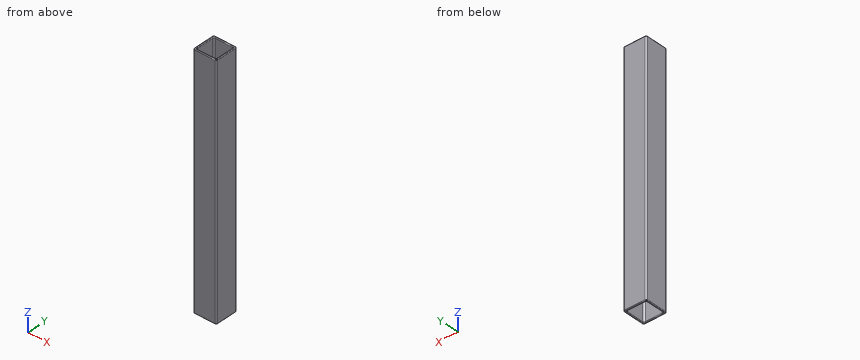
from build123d import *

# Parameters (mm, degrees)
BOSS_EXTRUDE1_DEPTH = 397
BOSS_EXTRUDE2_START = 0.678713738
BOSS_EXTRUDE2_DEPTH = 0.678713738
FILLET1_R           = 1


with BuildPart() as part:
    # Sketch1 → Boss-Extrude1 (new body)
    with BuildSketch(Plane.XY):
        with BuildLine():
            Line((2.54, 0), (35.56, 0))
            ThreePointArc((35.56, 0), (37.356051224, -0.743948776), (38.1, -2.54))
            Line((38.1, -2.54), (38.1, -35.56))
            ThreePointArc((38.1, -35.56), (37.356051224, -37.356051224), (35.56, -38.1))
            Line((35.56, -38.1), (2.54, -38.1))
            ThreePointArc((2.54, -38.1), (0.743948776, -37.356051224), (0, -35.56))
            Line((0, -35.56), (0, -2.54))
            ThreePointArc((0, -2.54), (0.743948776, -0.743948776), (2.54, 0))
        make_face()
        with BuildLine():
            Line((5.3086, -2.7686), (32.7914, -2.7686))
            ThreePointArc((32.7914, -2.7686), (34.587451224, -3.512548776), (35.3314, -5.3086))
            Line((35.3314, -5.3086), (35.3314, -32.7914))
            ThreePointArc((35.3314, -32.7914), (34.587451224, -34.587451224), (32.7914, -35.3314))
            Line((32.7914, -35.3314), (5.3086, -35.3314))
            ThreePointArc((5.3086, -35.3314), (3.512548776, -34.587451224), (2.7686, -32.7914))
            Line((2.7686, -32.7914), (2.7686, -5.3086))
            ThreePointArc((2.7686, -5.3086), (3.512548776, -3.512548776), (5.3086, -2.7686))
        make_face(mode=Mode.SUBTRACT)
    extrude(amount=BOSS_EXTRUDE1_DEPTH)

    # Sketch2 → Boss-Extrude2 (add)
    with BuildSketch(Plane(origin=(0, 0, 0), x_dir=(-1, 0, 0), z_dir=(0, 0, -1)).offset(BOSS_EXTRUDE2_START)):
        with BuildLine():
            Line((0, -35.56), (0, -2.54))
            ThreePointArc((0, -2.54), (-0.743948776, -0.743948776), (-2.54, 0))
            Line((-2.54, 0), (-35.56, 0))
            ThreePointArc((-35.56, 0), (-37.356051224, -0.743948776), (-38.1, -2.54))
            Line((-38.1, -2.54), (-38.1, -35.56))
            ThreePointArc((-38.1, -35.56), (-37.356051224, -37.356051224), (-35.56, -38.1))
            Line((-35.56, -38.1), (-2.54, -38.1))
            ThreePointArc((-2.54, -38.1), (-0.743948776, -37.356051224), (0, -35.56))
        make_face()
        with BuildLine():
            Line((-32.7914, -2.7686), (-5.3086, -2.7686))
            ThreePointArc((-5.3086, -2.7686), (-3.512548776, -3.512548776), (-2.7686, -5.3086))
            Line((-2.7686, -5.3086), (-2.7686, -32.7914))
            ThreePointArc((-2.7686, -32.7914), (-3.512548776, -34.587451224), (-5.3086, -35.3314))
            Line((-5.3086, -35.3314), (-32.7914, -35.3314))
            ThreePointArc((-32.7914, -35.3314), (-34.587451224, -34.587451224), (-35.3314, -32.7914))
            Line((-35.3314, -32.7914), (-35.3314, -5.3086))
            ThreePointArc((-35.3314, -5.3086), (-34.587451224, -3.512548776), (-32.7914, -2.7686))
        make_face(mode=Mode.SUBTRACT)
    extrude(amount=-BOSS_EXTRUDE2_DEPTH)

    # Fillet1
    fillet1_edges = [part.edges().sort_by_distance(p)[0] for p in [
        (37.356051224, -37.356051224, 397),
        (38.1, -19.05, 397),
        (37.356051224, -0.743948776, 397),
        (19.05, 0, 397),
        (0.743948776, -0.743948776, 397),
        (0, -19.05, 397),
        (3.512548776, -34.587451224, 397),
        (19.05, -35.3314, 397),
        (34.587451224, -34.587451224, 397),
        (35.3314, -19.05, 397),
        (34.587451224, -3.512548776, 397),
        (19.05, -2.7686, 397),
        (3.512548776, -3.512548776, 397),
        (2.7686, -19.05, 397),
        (0.743948776, -37.356051224, 397),
        (19.05, -2.7686, -0.678713738),
        (3.512548776, -3.512548776, -0.678713738),
        (2.7686, -19.05, -0.678713738),
        (3.512548776, -34.587451224, -0.678713738),
        (19.05, -35.3314, -0.678713738),
        (34.587451224, -34.587451224, -0.678713738),
        (35.3314, -19.05, -0.678713738),
        (34.587451224, -3.512548776, -0.678713738),
        (19.05, -38.1, -0.678713738),
        (0.743948776, -37.356051224, -0.678713738),
        (0, -19.05, -0.678713738),
        (0.743948776, -0.743948776, -0.678713738),
        (19.05, 0, -0.678713738),
        (37.356051224, -0.743948776, -0.678713738),
        (38.1, -19.05, -0.678713738),
        (37.356051224, -37.356051224, -0.678713738),
        (19.05, -38.1, 397),
    ]]
    fillet(fillet1_edges, radius=FILLET1_R)


solid = part.part
Work out the finished part from the listing and answer in its coordinate system (mm). Round coordinates to 2 decimals unless told otherwise and drop trailing zeros. Write each loop counter-clockwise with the first axis right and the second up, starting at its lowest first coordinate (ties: lowest second). Pieces come first, ordered by that corner, then holes. Notation, with made-up numbers: (20.5, 78.25) - (68.5, 78.25) arc R29 cw to (68.5, 114.25) - close; hole circle Ø11 at (24.25, 36.25). An arc over 180 degrees is marked (long way). Answer in a Markdown table with one row per item. Add a question column.
1. A cutting plane is placed at C-C, the plane x = 29.5. Determine the outline of the cut face in (y, z).
2. A cutting plane is placed at B-B, the plane z = 348.5. Determine the outline of the cut face in (x, y).
3. A cutting plane is placed at A-A, the plane y = -25.5. Determine the outline of the cut face in (x, z).
4. Find the intervals of material crossed by line 1 along X through (y, z) = (-8, 304); line 2 along Y through (x, z) = (9.5, 131); line 3 along Z through (x, y) = (2, -11), in increasing order. Write a range as from..to.
5. Given pin 1 (8 mm diameter, centred on x = 15.5, y = -7.5, fed in from +Z), flat-ended and moving along its own axis, determine where the tip first touches the part or whether it passes through.
Worked out:
| question | item | result |
|---|---|---|
| 1 | outline | (-38.1, 0.32) arc R1 ccw to (-37.1, -0.68) - (-36.33, -0.68) arc R1 ccw to (-35.33, 0.32) - (-35.33, 396) arc R1 ccw to (-36.33, 397) - (-37.1, 397) arc R1 ccw to (-38.1, 396) - close; (-2.77, 0.32) arc R1 ccw to (-1.77, -0.68) - (-1, -0.68) arc R1 ccw to (0, 0.32) - (0, 396) arc R1 ccw to (-1, 397) - (-1.77, 397) arc R1 ccw to (-2.77, 396) - close |
| 2 | outline | (0, -35.56) arc R2.54 ccw to (2.54, -38.1) - (35.56, -38.1) arc R2.54 ccw to (38.1, -35.56) - (38.1, -2.54) arc R2.54 ccw to (35.56, 0) - (2.54, 0) arc R2.54 ccw to (0, -2.54) - close; hole (2.77, -32.79) arc R2.54 ccw to (5.31, -35.33) - (32.79, -35.33) arc R2.54 ccw to (35.33, -32.79) - (35.33, -5.31) arc R2.54 ccw to (32.79, -2.77) - (5.31, -2.77) arc R2.54 ccw to (2.77, -5.31) - close |
| 3 | outline | (0, 0.32) arc R1 ccw to (1, -0.68) - (1.77, -0.68) arc R1 ccw to (2.77, 0.32) - (2.77, 396) arc R1 ccw to (1.77, 397) - (1, 397) arc R1 ccw to (0, 396) - close; (35.33, 0.32) arc R1 ccw to (36.33, -0.68) - (37.1, -0.68) arc R1 ccw to (38.1, 0.32) - (38.1, 396) arc R1 ccw to (37.1, 397) - (36.33, 397) arc R1 ccw to (35.33, 396) - close |
| 4 | line 1 | 0..2.77, 35.33..38.1 |
| 4 | line 2 | -38.1..-35.33, -2.77..0 |
| 4 | line 3 | -0.65..396.97 |
| 5 | pin 1 | through |
